Could you check a few things on this model? Use its own coordinates, in mm. A direction names the side the tool comes from. Coordinates: 2 decimals unless noted, no trailing zeros. Write each loop counter-clockwise with the first axis right and the second up, starting at its lowest first coordinate (ties: lowest second). Pieces come first, ordered by that corner, then holes.
```python
from build123d import *

# Parameters (mm, degrees)
SKETCH_1_W          = 20
SKETCH_1_H          = 34
EXTRUDE_1_DEPTH     = 5
SKETCH_2_W          = 20
SKETCH_2_H          = 3
EXTRUDE_2_DEPTH     = 5
EXTRUDE_3_DEPTH     = 5
FILLET_1_R          = 3
CUT_EXTRUDE_1_DEPTH = 2
SKETCH_7_R          = 1.6
CUT_EXTRUDE_2_DEPTH = 41.087864079
SKETCH_8_R          = 1.75
CUT_EXTRUDE_3_DEPTH = 41.087864079
CUT_EXTRUDE_5_DEPTH = 3.2
EXTRUDE_17_DEPTH    = 18
SKETCH_14_W         = 13
SKETCH_14_H         = 31
EXTRUDE_18_DEPTH    = 30
SKETCH_15_R         = 1.5
SKETCH_15_W         = 20.470707414
SKETCH_15_H         = 10.803453681
CUT_EXTRUDE_6_DEPTH = 61.249481326
SKETCH_16_W         = 16.444381011
SKETCH_16_H         = 28.281193961
CUT_EXTRUDE_7_DEPTH = 25
SKETCH_17_W         = 5
SKETCH_17_H         = 3
EXTRUDE_19_DEPTH    = 5
SKETCH_18_R         = 3
CUT_EXTRUDE_8_DEPTH = 3.5
SKETCH_19_W         = 4.5
SKETCH_19_H         = 27.2
EXTRUDE_20_DEPTH    = 25
SKETCH_20_W         = 8
SKETCH_20_H         = 13.2
CUT_EXTRUDE_9_DEPTH = 64.078600555


with BuildPart() as part:
    # 草图1 → 凸台-拉伸1 (new body)
    with BuildSketch(Plane.XY):
        with Locations((-10, 17)):
            Rectangle(SKETCH_1_W, SKETCH_1_H)
    extrude(amount=EXTRUDE_1_DEPTH)

    # 草图2 → 凸台-拉伸2 (add)
    with BuildSketch(Plane.XY.offset(5)):
        with Locations((-10, 32.5)):
            Rectangle(SKETCH_2_W, SKETCH_2_H)
        with Locations((-10, 1.5)):
            Rectangle(SKETCH_2_W, SKETCH_2_H)
    extrude(amount=EXTRUDE_2_DEPTH)

    # 草图4 → 凸台-拉伸3 (add)
    with BuildSketch(Plane(origin=(0, 0, 0), x_dir=(-1, 0, 0), z_dir=(0, 0, -1))):
        Polygon((0, 3), (0, 31), (-2.991740991, 31), (-20.640660029, 23.203556304), (-20.640660029, 10.796443696), (-2.991740991, 3), align=None)
        with BuildLine():
            ThreePointArc((-16, 15.25), (-17.75, 17), (-16, 18.75))
            Line((-16, 18.75), (-14, 18.75))
            ThreePointArc((-14, 18.75), (-12.25, 17), (-14, 15.25))
            Line((-14, 15.25), (-16, 15.25))
        make_face(mode=Mode.SUBTRACT)
    extrude(amount=-EXTRUDE_3_DEPTH)

    # 圆角1
    fillet_1_edges = [part.edges().sort_by_distance(p)[0] for p in [
        (20.640660029, 10.796443696, 2.5),
        (20.640660029, 23.203556304, 2.5),
    ]]
    fillet(fillet_1_edges, radius=FILLET_1_R)

    # 草图5 → 切除-拉伸1 (cut)
    with BuildSketch(Plane(origin=(0, 0, 0), x_dir=(-1, 0, 0), z_dir=(0, 0, -1))):
        with BuildLine():
            Line((-16, 20.25), (-13.505814151, 20.212208017))
            ThreePointArc((-13.505814151, 20.212208017), (-10.759461769, 16.75218561), (-14, 13.75))
            Line((-14, 13.75), (-16, 13.75))
            ThreePointArc((-16, 13.75), (-19.25, 17), (-16, 20.25))
        make_face()
    extrude(amount=-CUT_EXTRUDE_1_DEPTH, mode=Mode.SUBTRACT)

    # 草图7 → 切除-拉伸2 (cut, through all)
    with BuildSketch(Plane.XY.offset(5)):
        with Locations((-17.5, 22)):
            Circle(SKETCH_7_R)
        with Locations((-2.5, 22)):
            Circle(SKETCH_7_R)
        with Locations((-2.5, 12)):
            Circle(SKETCH_7_R)
        with Locations((-17.5, 12)):
            Circle(SKETCH_7_R)
    extrude(amount=-CUT_EXTRUDE_2_DEPTH, mode=Mode.SUBTRACT)

    # 草图8 → 切除-拉伸3 (cut, through all)
    with BuildSketch(Plane.XY.offset(5)):
        with Locations((-10, 17)):
            Circle(SKETCH_8_R)
    extrude(amount=-CUT_EXTRUDE_3_DEPTH, mode=Mode.SUBTRACT)

    # 草图9 → 切除-拉伸5 (cut)
    with BuildSketch(Plane(origin=(0, 0, 0), x_dir=(-1, 0, 0), z_dir=(0, 0, -1))):
        Polygon((11.668772273, 13.964345359), (13.463340173, 16.927371861), (11.7945679, 19.963026502), (8.331227727, 20.035654641), (6.536659827, 17.072628139), (8.2054321, 14.036973498), align=None)
    extrude(amount=-CUT_EXTRUDE_5_DEPTH, mode=Mode.SUBTRACT)

    # 草图12 → 凸台-拉伸17 (add)
    with BuildSketch(Plane.ZY.offset(20)):
        Polygon((10, 3), (5, 3), (5, 34), (0, 34), (0, 3), (0, 0), (10, 0), align=None)
    extrude(amount=EXTRUDE_17_DEPTH)

    # 草图14 → 凸台-拉伸18 (add)
    with BuildSketch(Plane.XY.offset(5)):
        with Locations((-31.5, 18.5)):
            Rectangle(SKETCH_14_W, SKETCH_14_H)
    extrude(amount=EXTRUDE_18_DEPTH)

    # 草图15 → 切除-拉伸6 (cut, through all)
    with BuildSketch(Plane.XZ.offset(-3)):
        with Locations((-33.2, 22)):
            Circle(SKETCH_15_R)
        with Locations((-32.765829074, 32.601726841)):
            Rectangle(SKETCH_15_W, SKETCH_15_H)
    extrude(amount=-CUT_EXTRUDE_6_DEPTH, mode=Mode.SUBTRACT)

    # 草图16 → 切除-拉伸7 (cut)
    with BuildSketch(Plane(origin=(0, 34, 0), x_dir=(1, 0, 0), z_dir=(0, 1, 0))):
        with Locations((-33.222190506, -13.05940302)):
            Rectangle(SKETCH_16_W, SKETCH_16_H)
    extrude(amount=-CUT_EXTRUDE_7_DEPTH, mode=Mode.SUBTRACT)

    # 草图17 → 凸台-拉伸19 (add)
    with BuildSketch(Plane.ZY.offset(20)):
        with Locations((7.5, 32.5)):
            Rectangle(SKETCH_17_W, SKETCH_17_H)
    extrude(amount=EXTRUDE_19_DEPTH)

    # 草图18 → 切除-拉伸8 (cut)
    with BuildSketch(Plane.XY.offset(5)):
        with Locations((-17.5, 22)):
            Circle(SKETCH_18_R)
        with Locations((-2.5, 22)):
            Circle(SKETCH_18_R)
        with Locations((-2.5, 12)):
            Circle(SKETCH_18_R)
        with Locations((-17.5, 12)):
            Circle(SKETCH_18_R)
    extrude(amount=-CUT_EXTRUDE_8_DEPTH, mode=Mode.SUBTRACT)

    # 草图19 → 凸台-拉伸20 (add)
    with BuildSketch(Plane(origin=(0, 9, 0), x_dir=(1, 0, 0), z_dir=(0, 1, 0))):
        with Locations((-27.25, -13.6)):
            Rectangle(SKETCH_19_W, SKETCH_19_H)
    extrude(amount=EXTRUDE_20_DEPTH)

    # 草图20 → 切除-拉伸9 (cut, through all)
    with BuildSketch(Plane(origin=(-25, 0, 0), x_dir=(0, 0, -1), z_dir=(1, 0, 0))):
        with Locations((-24.5, 19.6)):
            Rectangle(SKETCH_20_W, SKETCH_20_H)
        Polygon((-10, 34), (-27.2, 29.2), (-27.2, 34), align=None)
    extrude(amount=-CUT_EXTRUDE_9_DEPTH, mode=Mode.SUBTRACT)


solid = part.part
```
1. If we mould it in two halves opening along X, with no side actions, what happens to faces 1 (the face through (-12.553, 15.425, 1.578)), 2 (the face through (20.167, 22.866, 2.535)), 3 (the face through (2, 3, 2)), 4 (the face through (-1, 11, 1.5))? For each: pulls with the +X half, pulls with the -X half, needs draft (parallel to the pull), parting line crosses it, or undercut.
Verdict:
face 1: undercut
face 2: pulls with the +X half
face 3: needs draft
face 4: undercut
2. I want a section at D-D on y = 22. Please give me the cut outline in (x, z).
Verdict:
outline: (-29.5, 0) - (-19.1, 0) - (-19.1, 1.5) - (-20.5, 1.5) - (-20.5, 5) - (-25, 5) - (-25, 20.5) - (-29.5, 20.5) - close; (-15.9, 0) - (-4.1, 0) - (-4.1, 1.5) - (-5.5, 1.5) - (-5.5, 5) - (-14.5, 5) - (-14.5, 1.5) - (-15.9, 1.5) - close; (-0.9, 0) - (20.55, 0) - (20.55, 5) - (0.5, 5) - (0.5, 1.5) - (-0.9, 1.5) - close
3. I want a section at A-A on x = -33.2. Please give me the cut outline in (y, z).
Verdict:
outline: (0, 0) - (9, 0) - (9, 20.5) - (3, 20.5) - (3, 10) - (0, 10) - close; (3, 23.5) - (9, 23.5) - (9, 27.2) - (3, 27.2) - close
4. I want a section at C-C on z = 22. Please give me the cut outline in (x, y), plus the area to 3 significant figures.
Verdict:
outline: (-38, 3) - (-34.7, 3) - (-34.7, 9) - (-38, 9) - close; (-31.7, 3) - (-25, 3) - (-25, 13) - (-29.5, 13) - (-29.5, 9) - (-31.7, 9) - close; (-29.5, 26.2) - (-25, 26.2) - (-25, 30.65) - (-29.5, 30.65) - close
area: 98.0 mm2
5. On a 3-axis mill with a long thin cutter (end or side, diameter ignored), from which of +Z, -Z, +X, -X, +Y, -Y can I reach the whole of each face in a straight line? I mean faces 5 (the face through (-12.641, 18.424, 1.578)), 6 (the face through (0, 1, 5)), 7 (the face through (-2, 17, 5)), 8 (the face through (-27, 20, 20.5)), 9 (the face through (-4.9, 20.2, 3.3)). Say none if no direction works.
Verdict:
face 5: -Z
face 6: +Z, -Z, +X, -Y
face 7: +Z, +X
face 8: +Z, +X, -X
face 9: +Z
6. For pin 1 (1.5 mm diameter, centred on y = 5, z = 4, fed in from +X); pin 2 (2 mm diameter, centred on x = -26.5, z = 23, fed in from -Y); pin 3 (1.5 mm diameter, centred on x = -18, y = 28.5, fed in from +Z), each with a flat end and sliding along its axis, tell me the tip position at first contact or that it passes through.
Verdict:
pin 1: stops at x = 9.22
pin 2: stops at y = 3
pin 3: stops at z = 5
7. Please list where these lines run through material, in increasing order: line 1 along Y through (x, z) = (-17.5, 1); line 2 along Y through (x, z) = (-2.5, 3.5); line 3 along Z through (x, y) = (-33.2, 6.65).
Verdict:
line 1: y = 0 to 10.4, 13.6 to 20.4, 23.6 to 34
line 2: y = 0 to 9, 15 to 19, 25 to 34
line 3: z = 0 to 20.5, 23.5 to 27.2
8. I want a section at B-B on x = -17.5. Please give me the cut outline in (y, z).
Verdict:
outline: (0, 0) - (10.4, 0) - (10.4, 1.5) - (9, 1.5) - (9, 5) - (3, 5) - (3, 10) - (0, 10) - close; (13.6, 0) - (20.4, 0) - (20.4, 1.5) - (19, 1.5) - (19, 5) - (15, 5) - (15, 1.5) - (13.6, 1.5) - close; (23.6, 0) - (34, 0) - (34, 10) - (31, 10) - (31, 5) - (25, 5) - (25, 1.5) - (23.6, 1.5) - close
